Source: three-view drawing plus pictorial views. Frame: mm from the lowest corner of the part. A direction names the side the tool comes from. Give positions to 0.01 mm unless a question says otherwise; leave off trailing zeros. Order: outer loops, then holes, each group sorted by start corner. A loop starts at its lowest first (then second) coordinate and runs counter-clockwise, first axis right, second up. Notation, with made-up numbers: (-40, 28.25) - (-18, 28.25) arc R24 ccw to (-18, 38.25) - close; hole circle Ø2 at (8, 59.5). An arc over 180 degrees is marked (long way). Answer in a Markdown table with one row per item. Add a question column.
1. Mould query, pull axis Z, two halves, no side actions, for the marked faces 1, 2 and 3. Classes: released by +Z, released by -Z, zero draft, split by the parting line, or undercut.
2. Ray query, line 1 (Z direction, x = 5.5, y = 2.9); line 2 (Y direction, x = 5.5, z = 2.5); line 3 (Z direction, x = 7.75, y = 0.35). Return the intervals inside material, ascending. Write a range as [from, to].
3. Contact query for flat-ended pins moving along their axis: pin 1 (2 mm diameter, centred on y = 3, z = 9, fed in from +X); pin 2 (3 mm diameter, centred on x = 1.5, y = 1, fed in from -Z); pin 3 (2 mm diameter, centred on x = 7.5, y = 0.5, fed in from +Z). Output: stop coordinate, or through.
4. Access query for the marked faces 4 and 5. Directions: +Z, -Z, +X, -X, +Y, -Y. A direction counts if a zero-diameter tool reaches every point of the face in a straight line with its end or side. Return the directions, or none.
5. Section query C-C on z = 5.4. Return loops of the section in (x, y).
6. Section query B-B on x = 5.4. Return loops of the section in (y, z).
7. Section query A-A on y = 0.65. Return loops of the section in (x, z), and give its area (3 significant figures).
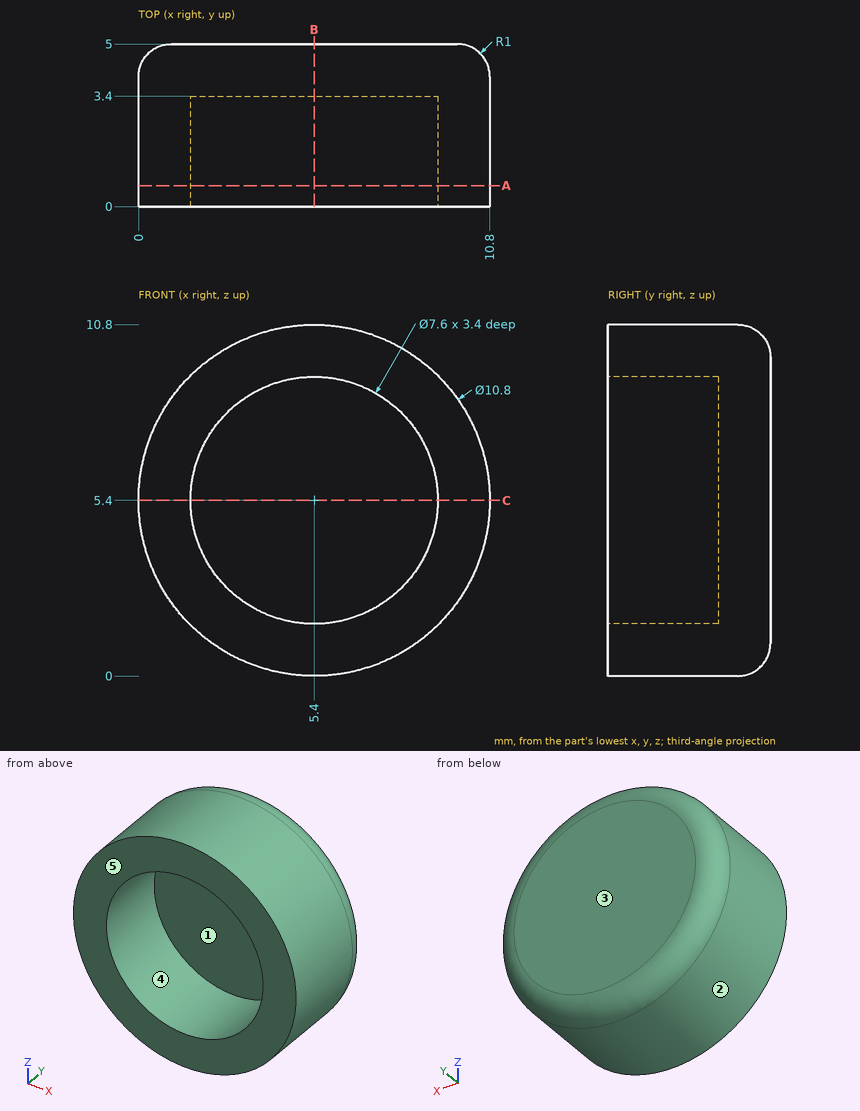
Answer:
| question | item | result |
|---|---|---|
| 1 | face 1 | undercut |
| 1 | face 2 | split by the parting line |
| 1 | face 3 | zero draft |
| 2 | line 1 | z = [0, 1.6], [9.2, 10.8] |
| 2 | line 2 | y = [3.4, 5] |
| 2 | line 3 | z = [0.54, 2.41], [8.39, 10.26] |
| 3 | pin 1 | stops at x = 10.13 |
| 3 | pin 2 | stops at z = 0.56 |
| 3 | pin 3 | stops at z = 10.69 |
| 4 | face 4 | -Y |
| 4 | face 5 | +Z, -Z, +X, -X, -Y |
| 5 | outline | (0, 0) - (1.6, 0) - (1.6, 3.4) - (9.2, 3.4) - (9.2, 0) - (10.8, 0) - (10.8, 4) arc R1 ccw to (9.8, 5) - (1, 5) arc R1 ccw to (0, 4) - close |
| 6 | outline | (0, 0) - (4, 0) arc R1 ccw to (5, 1) - (5, 9.8) arc R1 ccw to (4, 10.8) - (0, 10.8) - (0, 9.2) - (3.4, 9.2) - (3.4, 1.6) - (0, 1.6) - close |
| 7 | outline | circle Ø10.8 at (5.4, 5.4); hole circle Ø7.6 at (5.4, 5.4) |
| 7 | area | 46.2 mm² |
